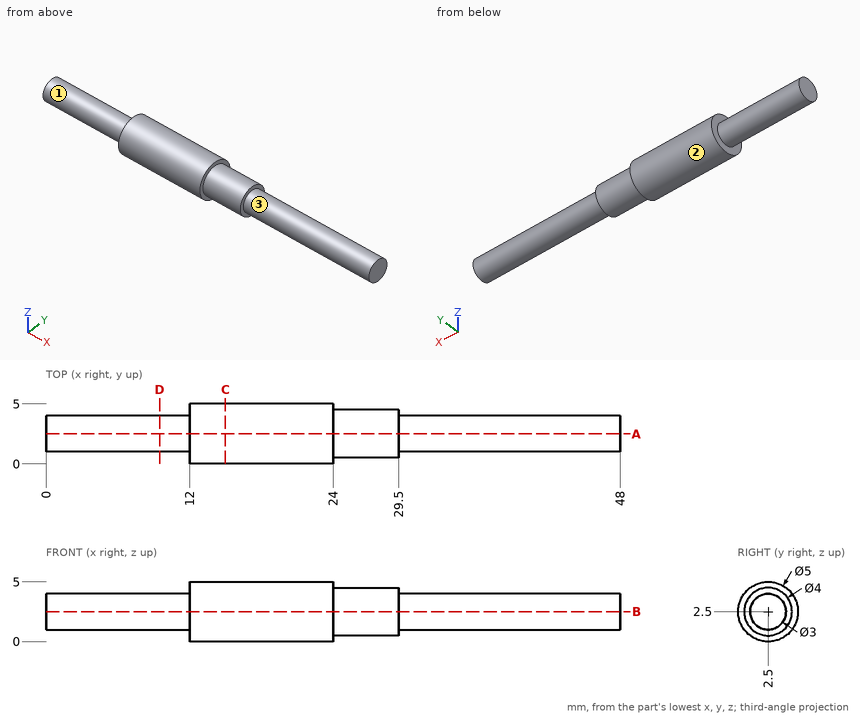
Answer from the drawing. Dimensions are ordinates in mm from the lowest x, y and z of the part. A direction names the side the tool comes from. Give positions to 0.01 mm unless a question says otherwise; leave off trailing zeros. Order: outer loops, then holes, each group sorted by start corner. A loop starts at its lowest first (then second) coordinate and runs counter-clockwise, first axis right, second up. Notation, with made-up numbers: (3, 29.25) - (48, 29.25) arc R30 cw to (48, 67.25) - close; hole circle Ø5 at (52.5, 45.5). An arc over 180 degrees is marked (long way). One line per item, written item: value. Start each with the question number.
1) A cutting plane is placed at A-A on y = 2.5. Give the vertices of the cut face in (x, z), then the cut area to 4 significant figures.
2) Find the intervals of material crossed by L1, parallel to X at y = 3.5, z = 3.65; L2, parallel to X at y = 0.9, z = 4.3; L3, parallel to Y at x = 2.5, z = 2.4, in increasing order.
3) Given pin 1 Ø3 at (x, z) = (34, 4.5) entering from -Y; pin 2 Ø1 at (x, y) = (38, 1) entering from -Z, each flat-ended and moving along its own axis, determine where each tip first touches the part or whether it passes through.
4) A tool of negligible diameter and unlimited length cuts with its end or side. For the marked faces 1, 2 and 3, from which of +Z, -Z, +X, -X, +Y, -Y can it reach the whole face along a straight path? Write none if from no direction.
5) A cutting plane is placed at D-D on x = 9.5. Give the vertices of the cut face in (y, z).
6) A cutting plane is placed at C-C on x = 15. Give the vertices of the cut face in (y, z), then the cut area to 3 significant figures.
Answer sheet:
1. outline: (0, 1) - (12, 1) - (12, 0) - (24, 0) - (24, 0.5) - (29.5, 0.5) - (29.5, 1) - (48, 1) - (48, 4) - (29.5, 4) - (29.5, 4.5) - (24, 4.5) - (24, 5) - (12, 5) - (12, 4) - (0, 4) - close
1. area: 173.5 mm2
2. L1: x = 12 to 29.5
2. L2: x = 12 to 24
2. L3: y = 1 to 4
3. pin 1: stops at y = 1.09
3. pin 2: stops at z = 1.38
4. face 1: -X
4. face 2: +X, -X
4. face 3: +X
5. outline: circle Ø3 at (2.5, 2.5)
6. outline: circle Ø5 at (2.5, 2.5)
6. area: 19.6 mm2
